Design review of the part shown in the three views and the two pictorial views. Dimensions are in mm from the part's minimum x, y and z. Coordinates: 2 decimals unless noted, no trailing zeros. Write each loop counter-clockwise with the first axis right and the second up, starting at its lowest first coordinate (ties: lowest second). Pieces come first, ordered by that corner, then holes. Notation, with made-up numbers: (61, -2.5) - (81, -2.5) arc R24 ccw to (81, 32.5) - close; hole circle Ø8 at (77, -9). An arc over 180 degrees is marked (long way). Answer as CSV lines item,"result". Start each with the question number.
Q1. We need section B-B (z = 1.65). Write out the cut boundary in (x, y).
Q2. We need section A-A (y = 5). Write out the cut boundary in (x, z).
Q3. For line 1 along Y through (x, z) = (195, 2.15); line 2 along X through (y, z) = (3.5, 2.9); line 3 along Y through (x, z) = (13, 1.35), list the stretches that pass through material, from the lowest coordinate up. Write a range as [from, to].
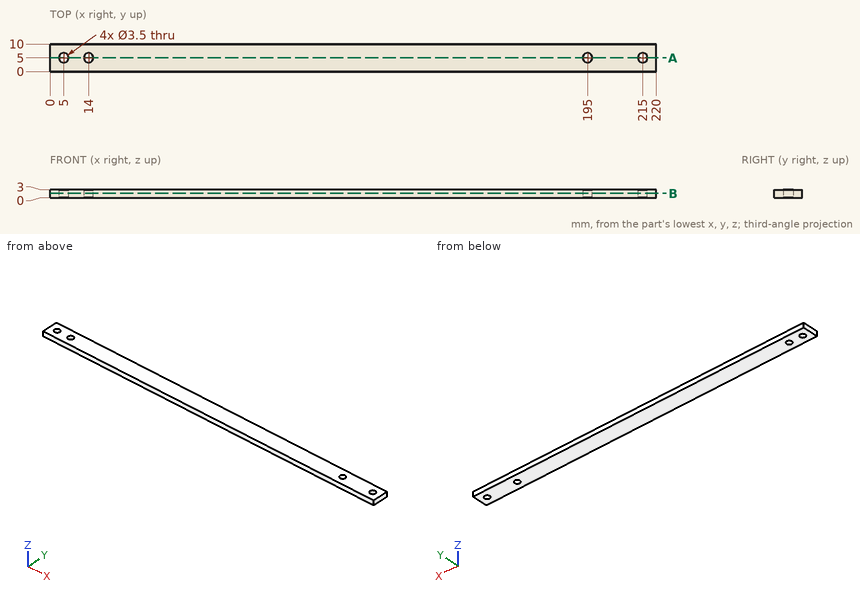
Results list:
1,outline,"(0, 0) - (220, 0) - (220, 10) - (0, 10) - close; hole circle Ø3.5 at (5, 5); hole circle Ø3.5 at (14, 5); hole circle Ø3.5 at (195, 5); hole circle Ø3.5 at (215, 5)"
2,outline,"(0, 0) - (3.25, 0) - (3.25, 3) - (0, 3) - close; (6.75, 0) - (12.25, 0) - (12.25, 3) - (6.75, 3) - close; (15.75, 0) - (193.25, 0) - (193.25, 3) - (15.75, 3) - close; (196.75, 0) - (213.25, 0) - (213.25, 3) - (196.75, 3) - close; (216.75, 0) - (220, 0) - (220, 3) - (216.75, 3) - close"
3,line 1,"y = [0, 3.25], [6.75, 10]"
3,line 2,"x = [0, 4.1], [5.9, 13.1], [14.9, 194.1], [195.9, 214.1], [215.9, 220]"
3,line 3,"y = [0, 3.56], [6.44, 10]"
